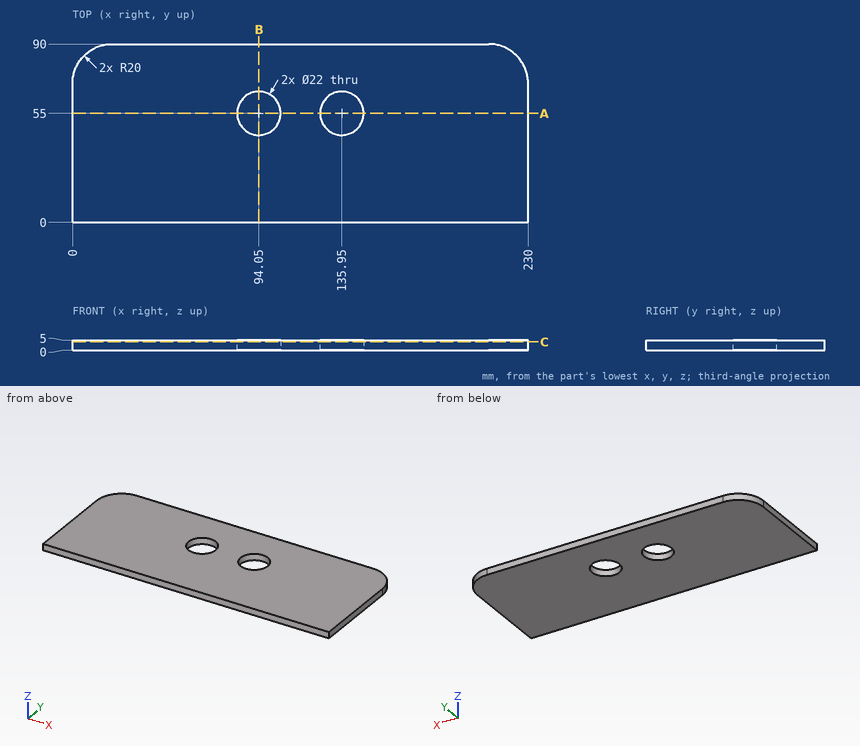
Input: dimensioned drawing with shaded views. Units: mm. Origin: part minimum x, y, z. Give positions to 0.01 mm unless a question says otherwise; leave off trailing zeros. Write each loop counter-clockwise with the first axis right and the second up, starting at its lowest first coordinate (ties: lowest second). Pieces come first, ordered by that corner, then holes.
Q1. Section A-A, the plane y = 55. Output: boundary loops of the cut face in (x, z), plus the area to 3 significant figures.
Q2. Section B-B, the plane x = 94.05. Output: boundary loops of the cut face in (y, z).
Q3. Section C-C, the plane z = 4.15. Output: boundary loops of the cut face in (x, y), plus the area to 3 significant figures.
Q4. First-contact query: P1, Ø3, axis at y = 50.5, z = 3, coming from the -X side; P2, Ø20, axis at x = 135.95, y = 55, coming from the +Z side. Flat tips, straight axial feed; report the tip coordinate or a pass-through.
Q5. Material intervals for probe 1 along Y at (x, z) = (135.95, 2.7); probe 2 along X at (y, z) = (48, 4.65); probe 3 along X at (y, z) = (47, 4.45), sorted ascending.
Filled in:
1. outline: (0, 0) - (83.05, 0) - (83.05, 5) - (0, 5) - close; (105.05, 0) - (124.95, 0) - (124.95, 5) - (105.05, 5) - close; (146.95, 0) - (230, 0) - (230, 5) - (146.95, 5) - close
1. area: 930 mm2
2. outline: (0, 0) - (44, 0) - (44, 5) - (0, 5) - close; (66, 0) - (90, 0) - (90, 5) - (66, 5) - close
3. outline: (0, 0) - (230, 0) - (230, 70) arc R20 ccw to (210, 90) - (20, 90) arc R20 ccw to (0, 70) - close; hole circle Ø22 at (94.05, 55); hole circle Ø22 at (135.95, 55)
3. area: 19,800 mm2
4. P1: stops at x = 0
4. P2: passes through
5. probe 1: y = 0 to 44, 66 to 90
5. probe 2: x = 0 to 85.56, 102.54 to 127.46, 144.44 to 230
5. probe 3: x = 0 to 86.5, 101.6 to 128.4, 143.5 to 230
